The model under review builds one solid part; all positions refer to its coordinate system, in mm. Face numbers are marked on the shaded views. A direction names the side the tool comes from. Round coordinates to 2 decimals unless told otherwise and drop trailing zeros. Loops run counter-clockwise (first coordinate to the right, second up) from the corner with the lowest first, then second, coordinate; pieces in that order, holes last. Notation, with made-up numbers: M 53.25,23.25 L 63.25,23.25 A30 ccw 63.25,50.25 Z; hole C -21,52.5 d9. An arc over 180 degrees is marked long. Return JSON: item names as keys, results as strings. Group by question number.
Q1. For the marked faces 5 and 6, list the 3-axis set-ups (+Z, -Z, +X, -X, +Y, -Y) from which the entire face can be reached by the end or side of a thin tool; tool diameter is ignored.
Q2. Consider section B-B (x = 13.25). State the section outline as (y, z) points.
Q3. Consider section C-C (y = 12). State the section outline as (x, z) points, and give its area (3 significant figures).
Q4. Clearance check with flat-ended pins moving along their axes: pin 1 Ø4.5 at (x, y) = (8.89, 4.445) entering from +Z; pin 2 Ø0.7 at (x, z) = (7, 1.5) entering from -Y. State where each tip first meets the part, or that it passes through.
Q5. To check wall thickness, follow line 1 along X through (y, z) = (4.5, 1.75); line 2 along Z through (x, y) = (4.75, 5.5); line 3 along Y through (x, z) = (8.89, 0.35). State the ranges of each line that lie inside material, in increasing order.
Q6. Draft analysis for pull direction X (two halves, no side actions). For the marked faces 1, 2, 3 and 4, state which applies: pulls with the +X half, pulls with the -X half, needs draft (parallel to the pull), parting line crosses it, or undercut.
Q7. Consider section A-A (x = 8.89). State the section outline as (y, z) points, and give its area (3 significant figures).
from build123d import *

# Parameters (mm, degrees)
F0_W     = 17.78
F0_H     = 12.7
F0_R     = 2.4892
F1_DEPTH = 2.54
F2_W     = 17.272
F2_H     = 1.397
F3_DEPTH = 8.89
F5_DEPTH = 17.78
F6_DEPTH = 25.4


with BuildPart() as f1:
    # F0 (on Top) → F1 (new body)
    with BuildSketch(Plane.XY):
        with Locations((8.89, 6.35)):
            Rectangle(F0_W, F0_H)
        with Locations((8.89, 4.445)):
            Circle(F0_R, mode=Mode.SUBTRACT)
    extrude(amount=F1_DEPTH)

    # F2 (on face) → F3 (cut)
    with BuildSketch(Plane.XZ):
        with Locations((8.89, 1.27)):
            Rectangle(F2_W, F2_H)
    extrude(amount=-F3_DEPTH, mode=Mode.SUBTRACT)

    # F4 (on face) → F5 (join)
    with BuildSketch(Plane(origin=(0, 0, 0), x_dir=(0, -1, 0), z_dir=(-1, 0, 0))):
        with BuildLine():
            Line((-12.7, 2.159), (-12.7, 2.54))
            ThreePointArc((-12.7, 2.54), (-13.97, 1.27), (-12.7, 0))
            Line((-12.7, 0), (-12.7, 0.381))
            ThreePointArc((-12.7, 0.381), (-13.589, 1.27), (-12.7, 2.159))
        make_face()
    extrude(amount=-F5_DEPTH)

    # F4 (on face) → F6 (cut)
    with BuildSketch(Plane(origin=(0, 0, 0), x_dir=(0, -1, 0), z_dir=(-1, 0, 0))):
        with BuildLine():
            ThreePointArc((-11.811, 1.27), (-12.071382, 1.898618), (-12.7, 2.159))
            Line((-12.7, 2.159), (-12.7, 0.381))
            ThreePointArc((-12.7, 0.381), (-12.071382, 0.641382), (-11.811, 1.27))
        make_face()
    extrude(amount=-F6_DEPTH, mode=Mode.SUBTRACT)


solid = f1.part
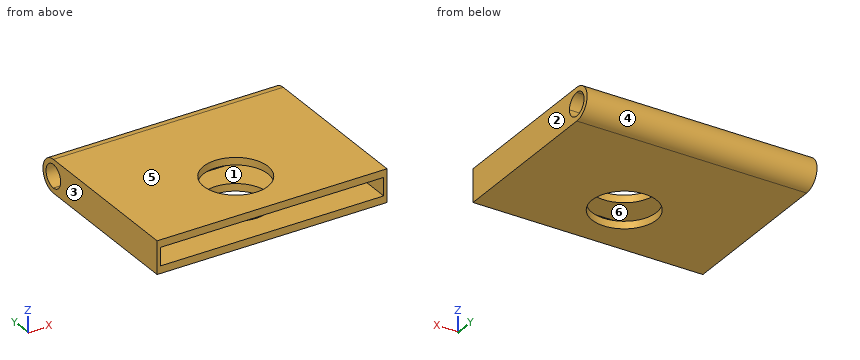
Values:
{
 "1": {"face 5": "+Z, +X, -X, +Y, -Y", "face 6": "-Y"},
 "2": {"outline": "M 0,0 L 12.7,0 A1.27 ccw 12.7,2.54 L 0,2.54 L 0,1.97 L 8.89,1.97 L 8.89,0.57 L 0,0.57 Z; hole C 12.7,1.27 d1.78"},
 "3": {"outline": "M 0,0 L 17.78,0 L 17.78,0.72 L 0,0.72 Z; M 0,1.82 L 17.78,1.82 L 17.78,2.54 L 0,2.54 Z", "area": "25.7 mm2"},
 "4": {"pin 1": "passes through", "pin 2": "stops at y = 8.89"},
 "5": {"line 1": "x = 0 to 0.25, 17.53 to 17.78", "line 2": "z = 0 to 0.57, 1.97 to 2.54", "line 3": "y = 0 to 1.96, 6.93 to 13.58"},
 "6": {"face 1": "undercut", "face 2": "pulls with the +X half", "face 3": "pulls with the -X half", "face 4": "needs draft"},
 "7": {"outline": "M 0,0 L 1.96,0 L 1.96,0.57 L 0,0.57 Z; M 0,1.97 L 1.96,1.97 L 1.96,2.54 L 0,2.54 Z; M 6.93,0 L 12.7,0 A1.27 ccw 12.7,2.54 L 6.93,2.54 L 6.93,1.97 L 8.89,1.97 L 8.89,0.57 L 6.93,0.57 Z; hole C 12.7,1.27 d1.78", "area": "14.2 mm2"}
}
